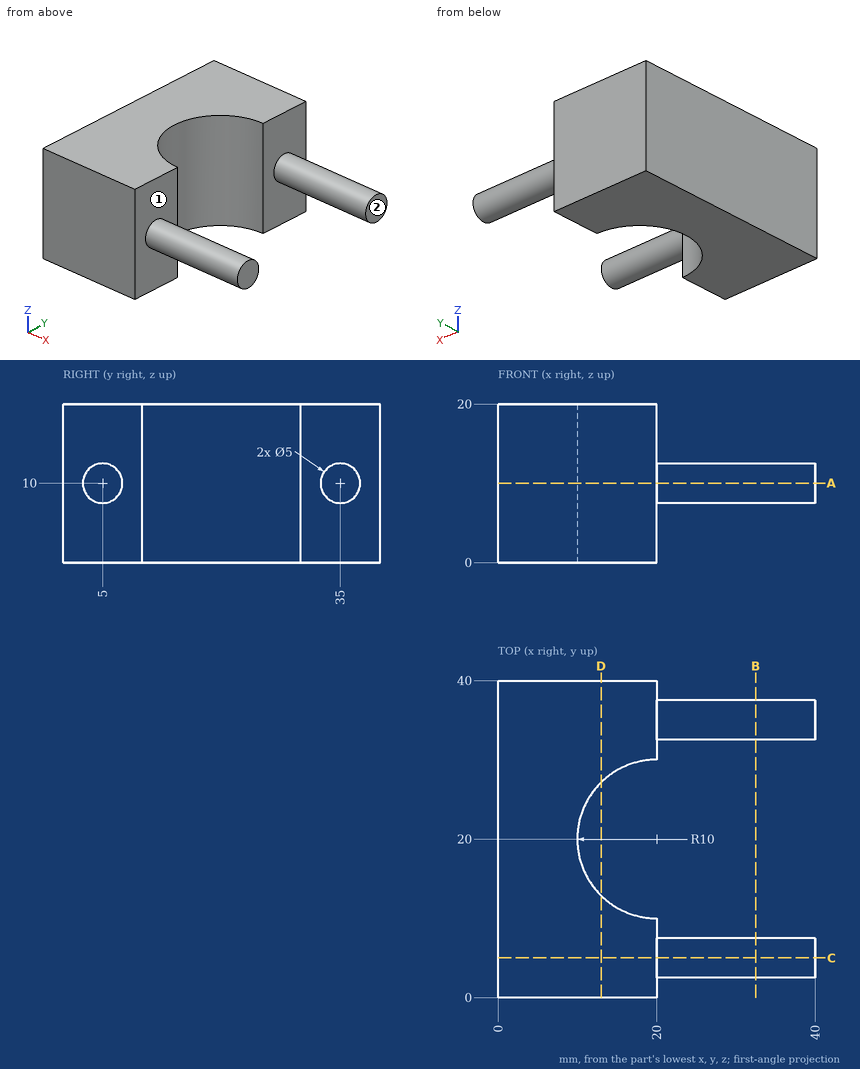
Geometry: see drawing. Coordinates: mm, zero at the bounding-box minimum. A direction names the side the tool comes from. Give positions to 0.01 mm unless a question says otherwise; leave off trailing zeros. Order: outer loops, then holes, each group sorted by start corner. A loop starts at its lowest first (then second) coordinate and runs counter-clockwise, first axis right, second up. Notation, with made-up numbers: (52.25, 16.5) -> (81.25, 16.5) arc R26 cw to (81.25, 36.5) -> close; hole circle Ø10 at (4.5, -0.5). An arc over 180 degrees is marked (long way). Write each question's results on one line, items separated by ' | '.
1) Cut plane D-D (x = 13). Output: boundary loops of the cut face in (y, z).
Geometry says:
outline: (0, 0) -> (12.86, 0) -> (12.86, 20) -> (0, 20) -> close; (27.14, 0) -> (40, 0) -> (40, 20) -> (27.14, 20) -> close
2) Set-up query: the marked faces 1 and 2. Return all of +Z, -Z, +X, -X, +Y, -Y with unobstructed straight access to the full face (end or side cutting, diameter ignored); none if empty.
Geometry says:
face 1: +X | face 2: +Z, -Z, +X, +Y, -Y
3) First-contact query: pin 1 Ø10 at (y, z) = (35, 17.5) entering from -X; pin 2 Ø2 at (y, z) = (17.5, 10.5) entering from +X; pin 3 Ø10 at (y, z) = (21.5, 17) entering from +X. Flat tips, straight axial feed; report the tip coordinate or a pass-through.
Geometry says:
pin 1: stops at x = 0 | pin 2: stops at x = 10.63 | pin 3: stops at x = 12.4
4) Cut plane A-A (z = 10). Output: boundary loops of the cut face in (x, y).
Geometry says:
outline: (0, 0) -> (20, 0) -> (20, 2.5) -> (40, 2.5) -> (40, 7.5) -> (20, 7.5) -> (20, 10) arc R10 cw to (20, 30) -> (20, 32.5) -> (40, 32.5) -> (40, 37.5) -> (20, 37.5) -> (20, 40) -> (0, 40) -> close
5) Cut plane B-B (x = 32.5). Output: boundary loops of the cut face in (y, z).
Geometry says:
outline: circle Ø5 at (5, 10); circle Ø5 at (35, 10)
6) Cut plane C-C (y = 5). Output: boundary loops of the cut face in (x, z), and give its area (3 significant figures).
Geometry says:
outline: (0, 0) -> (20, 0) -> (20, 7.5) -> (40, 7.5) -> (40, 12.5) -> (20, 12.5) -> (20, 20) -> (0, 20) -> close | area: 500 mm²
7) Line query: line 1 along X through (y, z) = (35, 13); line 2 along Y through (x, z) = (15.5, 2.5); line 3 along X through (y, z) = (20, 7.5). Output: solid intervals per line, ascending.
Geometry says:
line 1: x = 0 to 20 | line 2: y = 0 to 11.07, 28.93 to 40 | line 3: x = 0 to 10
